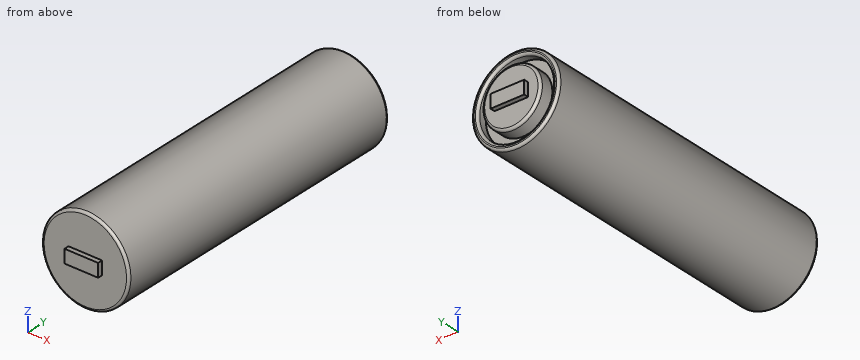
from build123d import *

# Parameters (mm, degrees)
SKETCH_1_R          = 9
EXTRUDE_1_DEPTH     = 65
SKETCH_2_R          = 7.75
SKETCH_2_R_2        = 6
CUT_EXTRUDE_1_DEPTH = 2
EXTRUDE_START       = 1
SKETCH_4_R          = 6
EXTRUDE_3_DEPTH     = 1
FILLET_1_R          = 0.5
SKETCH_3_W          = 6.932919868
SKETCH_3_H          = 2.75170262
EXTRUDE_910_DEPTH   = 1
SKETCH_5_W          = 6.932919868
SKETCH_5_H          = 2.75170262
EXTRUDE_1061_DEPTH  = 1


with BuildPart() as part:
    # 草图1 → 凸台-拉伸1 (new body)
    with BuildSketch(Plane(origin=(0, 0, 0), x_dir=(1, 0, 0), z_dir=(0, 1, 0))):
        with Locations(Location((0, 0, 0), (0, 0, 270))):
            Circle(SKETCH_1_R)
    extrude(amount=EXTRUDE_1_DEPTH)

    # 草图2 → 切除-拉伸1 (cut)
    with BuildSketch(Plane(origin=(0, 65, 0), x_dir=(1, 0, 0), z_dir=(0, 1, 0))):
        with Locations(Location((0, 0, 0), (0, 0, 270))):
            Circle(SKETCH_2_R)
        with Locations(Location((0, 0, 0), (0, 0, 270))):
            Circle(SKETCH_2_R_2, mode=Mode.SUBTRACT)
    extrude(amount=-CUT_EXTRUDE_1_DEPTH, mode=Mode.SUBTRACT)

    # 草图4 → 凸台-拉伸3 (add)
    with BuildSketch(Plane(origin=(0, 65, 0), x_dir=(1, 0, 0), z_dir=(0, 1, 0)).offset(EXTRUDE_START)):
        with Locations(Location((0, 0, 0), (0, 0, 270))):
            Circle(SKETCH_4_R)
    extrude(amount=-EXTRUDE_3_DEPTH)

    # 圆角1
    fillet_1_edges = [part.edges().sort_by_distance(p)[0] for p in [
        (0, 66, -6),
        (0, 0, -9),
        (0, 65, -9),
        (0, 65, -7.75),
    ]]
    fillet(fillet_1_edges, radius=FILLET_1_R)

    # 草图3 → Extrude 910 (add)
    with BuildSketch(Plane.XZ):
        Rectangle(SKETCH_3_W, SKETCH_3_H)
    extrude(amount=EXTRUDE_910_DEPTH)

    # 草图5 → Extrude 1061 (add)
    with BuildSketch(Plane(origin=(0, 66, 0), x_dir=(1, 0, 0), z_dir=(0, 1, 0))):
        Rectangle(SKETCH_5_W, SKETCH_5_H)
    extrude(amount=EXTRUDE_1061_DEPTH)


solid = part.part
Check sheet for the modelled part. Datum: model origin and axes. Units: mm. Round coordinates to 2 decimals unless told otherwise and drop trailing zeros. Write each loop counter-clockwise with the first axis right and the second up, starting at its lowest first coordinate (ties: lowest second). Pieces come first, ordered by that corner, then holes. Notation, with made-up numbers: (70.25, -39) -> (96.25, -39) arc R23 cw to (96.25, -14) -> close; hole circle Ø1 at (-29, 10). An arc over 180 degrees is marked (long way). Answer as CSV lines item,"result". Start each with the question number.
1) Section check B-B on z = 0. Enter the section's corners in (x, y), and give its area (3 significant figures).
2) Material ranges on line 1 (X direction, y = 63.85, z = 0); line 2 (Y direction, x = -5, z = 4.5); line 3 (Y direction, x = -4.5, z = 2.25), recorded low to high. Write a range as from..to.
3) Go/stop test with flat-tipped pins: P1, Ø1, axis at x = -7, y = 44, coming from the -Z side; P2, Ø3, axis at x = 7, y = 32, coming from the -Z side; P3, Ø1.5, axis at x = -4, y = 8.5, coming from the +Z side. Record where each tip stops, or that it passes through.
4) Section check C-C on y = 58. Enter the section's corners in (x, z), and give its area (3 significant figures).
5) Section check A-A on x = 0. Enter the section's corners in (y, z).
Found:
1,outline,"(-9, 0.5) arc R0.5 ccw to (-8.5, 0) -> (-3.47, 0) -> (-3.47, -1) -> (3.47, -1) -> (3.47, 0) -> (8.5, 0) arc R0.5 ccw to (9, 0.5) -> (9, 64.5) arc R0.5 ccw to (8.5, 65) -> (8.25, 65) arc R0.5 ccw to (7.75, 64.5) -> (7.75, 63) -> (6, 63) -> (6, 65.5) arc R0.5 ccw to (5.5, 66) -> (3.47, 66) -> (3.47, 67) -> (-3.47, 67) -> (-3.47, 66) -> (-5.5, 66) arc R0.5 ccw to (-6, 65.5) -> (-6, 63) -> (-7.75, 63) -> (-7.75, 64.5) arc R0.5 ccw to (-8.25, 65) -> (-8.5, 65) arc R0.5 ccw to (-9, 64.5) -> close"
1,area,"1,190 mm^2"
2,line 1,"x = -9..-7.75, -6..6, 7.75..9"
2,line 2,"y = 0..63"
2,line 3,"y = 0..66"
3,P1,"stops at z = -6.22"
3,P2,"stops at z = -7.12"
3,P3,"stops at z = 8.39"
4,outline,"circle Ø18 at (0, 0)"
4,area,"254 mm^2"
5,outline,"(-1, -1.38) -> (0, -1.38) -> (0, -8.5) arc R0.5 ccw to (0.5, -9) -> (64.5, -9) arc R0.5 ccw to (65, -8.5) -> (65, -8.25) arc R0.5 ccw to (64.5, -7.75) -> (63, -7.75) -> (63, -6) -> (65.5, -6) arc R0.5 ccw to (66, -5.5) -> (66, -1.38) -> (67, -1.38) -> (67, 1.38) -> (66, 1.38) -> (66, 5.5) arc R0.5 ccw to (65.5, 6) -> (63, 6) -> (63, 7.75) -> (64.5, 7.75) arc R0.5 ccw to (65, 8.25) -> (65, 8.5) arc R0.5 ccw to (64.5, 9) -> (0.5, 9) arc R0.5 ccw to (0, 8.5) -> (0, 1.38) -> (-1, 1.38) -> close"
